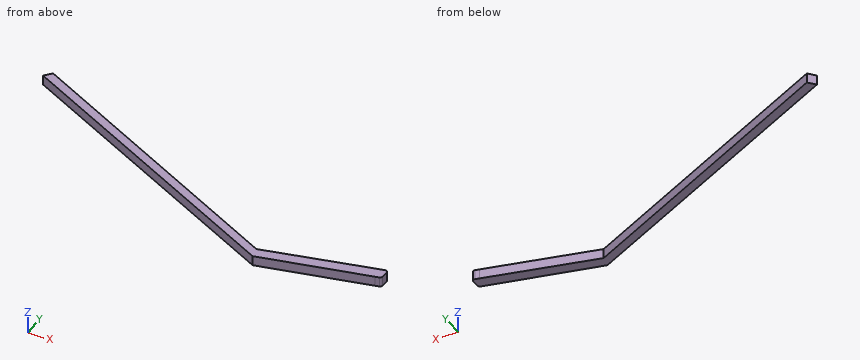
```python
from build123d import *

# Parameters (mm, degrees)
EXTRUDE_1_DEPTH = 2


with BuildPart() as part:
    # 스케치1 → 보스-돌출1 (new body)
    with BuildSketch(Plane.XY):
        with BuildLine():
            Line((-103.31355612, 14.450417953), (-102.023901871, 15.926355594))
            Line((-102.023901871, 15.926355594), (-42.998303114, -14.389807184))
            Line((-42.998303114, -14.389807184), (-20.223148332, -9.012633862))
            Line((-20.223148332, -9.012633862), (-19.43297603, -8.834019872))
            ThreePointArc((-19.43297603, -8.834019872), (-19.009782772, -8.930396085), (-18.821401864, -9.321412122))
            Line((-18.821401864, -9.321412122), (-18.821401864, -10.860213775))
            ThreePointArc((-18.821401864, -10.860213775), (-18.930385827, -11.171832867), (-19.209827698, -11.347606025))
            Line((-19.209827698, -11.347606025), (-20, -11.526220015))
            Line((-20, -11.526220015), (-42.500319357, -16.677300826))
            Line((-42.500319357, -16.677300826), (-103.31355612, 14.450417953))
        make_face()
    extrude(amount=EXTRUDE_1_DEPTH)


solid = part.part
```
Model file for the job. Use its own axes, mm. Round coordinates to 2 decimals unless told otherwise and drop trailing zeros. Loops run counter-clockwise (first coordinate to the right, second up) from the corner with the lowest first, then second, coordinate; pieces in that order, holes last. Notation, with made-up numbers: M 2,-14.5 L 19,-14.5 A21 cw 19,-0.5 Z; hole C 21.25,62 d11. An arc over 180 degrees is marked long. Put each result on its own line as item: value. Start each with the question number.
Item 1: Cut at C-C (x = -77.5). List the corners of the cut face in (y, z).
Item 2: Drill centre lines: line 1 along X through (y, z) = (8, 0.1); line 2 along Y through (x, z) = (-89, 1.1); line 3 along X through (y, z) = (-7, 0.9). Where is each one in solid material? Low to high.
Item 3: Cut at B-B (y = -13). List the corners of the cut face in (x, z), then the cut area to 3 significant figures.
Item 4: Cut at A-A (z = 0.3). List the corners of the cut face in (x, y), then the cut area to 3 significant figures.
Item 5: Cut at D-D (y = -0.5). List the corners of the cut face in (x, z).
Answer block:
1. outline: M 1.24,0 L 3.33,0 L 3.33,2 L 1.24,2 Z
2. line 1: -90.71 to -86.59
2. line 2: 7.12 to 9.24
2. line 3: -61.41 to -57.39
3. outline: M -49.68,0 L -45.7,0 L -45.7,2 L -49.68,2 Z; M -37.11,0 L -26.44,0 L -26.44,2 L -37.11,2 Z
3. area: 29.3 mm2
4. outline: M -103.31,14.45 L -42.5,-16.68 L -20,-11.53 L -19.21,-11.35 A0.5 ccw -18.82,-10.86 L -18.82,-9.32 A0.5 ccw -19.43,-8.83 L -20.22,-9.01 L -43,-14.39 L -102.02,15.93 Z
4. area: 184 mm2
5. outline: M -74.11,0 L -70.04,0 L -70.04,2 L -74.11,2 Z
